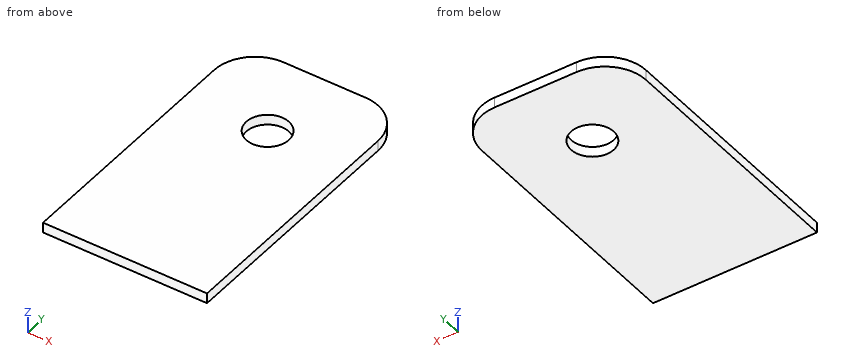
from build123d import *

# Parameters (mm, degrees)
SKETCH1_W               = 25.4
SKETCH1_H               = 31.75
BOSS_EXTRUDE1_DEPTH     = 1.5875
CUT_EXTRUDE1_DEPTH      = 35.232625611
CUT_EXTRUDE1_DEPTH_BACK = 35.232625611
SKETCH2_R               = 3.302
FILLET1_R               = 6.35
SKETCH3_W               = 25.4
SKETCH3_H               = 12.7
BOSS_EXTRUDE2_DEPTH     = 1.5875


with BuildPart() as part:
    # Sketch1 → Boss-Extrude1 (new body)
    with BuildSketch(Plane.XY):
        with Locations((0, 15.875)):
            Rectangle(SKETCH1_W, SKETCH1_H)
    extrude(amount=BOSS_EXTRUDE1_DEPTH)

    # Sketch2 → Cut-Extrude1 (cut, two sides: drawn at the far end of the back side and taken through both)
    with BuildSketch(Plane.XY.offset(1.5875).offset(-CUT_EXTRUDE1_DEPTH_BACK)):
        with Locations((0, 19.05)):
            Circle(SKETCH2_R)
    extrude(amount=CUT_EXTRUDE1_DEPTH + CUT_EXTRUDE1_DEPTH_BACK, mode=Mode.SUBTRACT)

    # Fillet1
    fillet1_edges = [part.edges().sort_by_distance(p)[0] for p in [
        (-12.7, 31.75, 0.79375),
        (12.7, 31.75, 0.79375),
    ]]
    fillet(fillet1_edges, radius=FILLET1_R)

    # Sketch3 → Boss-Extrude2 (add)
    with BuildSketch(Plane(origin=(0, 0, 0), x_dir=(-1, 0, 0), z_dir=(0, 0, -1))):
        with Locations((0, -6.35)):
            Rectangle(SKETCH3_W, SKETCH3_H)
    extrude(amount=-BOSS_EXTRUDE2_DEPTH)


solid = part.part
Work out the finished part from the listing and answer in its coordinate system (mm). Coordinates: 2 decimals unless noted, no trailing zeros. Write each loop counter-clockwise with the first axis right and the second up, starting at its lowest first coordinate (ties: lowest second). Pieces come first, ordered by that corner, then holes. Notation, with made-up numbers: (24.5, 66) - (75.5, 66) arc R35 cw to (75.5, 98) - close; hole circle Ø8 at (7.25, 64.25). An arc over 180 degrees is marked (long way). One line per question, with ' | ' between items.
1) Find section C-C, the plane x = 0. Determine the outline of the cut face in (y, z).
Checks:
outline: (-12.7, 0) - (15.75, 0) - (15.75, 1.59) - (-12.7, 1.59) - close; (22.35, 0) - (31.75, 0) - (31.75, 1.59) - (22.35, 1.59) - close
2) Find section A-A, the plane z = 0.75. Determine the outline of the cut face in (x, y), and give its area (3 significant figures).
Checks:
outline: (-12.7, -12.7) - (12.7, -12.7) - (12.7, 25.4) arc R6.35 ccw to (6.35, 31.75) - (-6.35, 31.75) arc R6.35 ccw to (-12.7, 25.4) - close; hole circle Ø6.6 at (0, 19.05) | area: 1,080 mm2
3) Consider probe 1 along Y at (x, z) = (0.25, 0.25); probe 2 along X at (y, z) = (19.05, 0.4); probe 3 along Y at (x, z) = (0, 1.2). Determine where each line is inside the solid, lowest interval first. Write a range as [from, to].
Checks:
probe 1: [-12.7, 15.76], [22.34, 31.75] | probe 2: [-12.7, -3.3], [3.3, 12.7] | probe 3: [-12.7, 15.75], [22.35, 31.75]
4) Find section B-B, the plane y = 19.05. Determine the outline of the cut face in (x, z).
Checks:
outline: (-12.7, 0) - (-3.3, 0) - (-3.3, 1.59) - (-12.7, 1.59) - close; (3.3, 0) - (12.7, 0) - (12.7, 1.59) - (3.3, 1.59) - close
5) Find section D-D, the plane y = 29. Determine the outline of the cut face in (x, z), and give its area (3 significant figures).
Checks:
outline: (-11.58, 0) - (11.58, 0) - (11.58, 1.59) - (-11.58, 1.59) - close | area: 36.8 mm2
